Input: part model. Units: mm. Frame: model coordinates. Give positions to 0.01 mm unless a question says otherwise; leave off trailing zeros. Loops run counter-clockwise (first coordinate to the right, second up) from the corner with the lowest first, then second, coordinate; pieces in that order, holes last. Notation, with made-up numbers: (67.25, 79) - (79.25, 79) arc R14 cw to (79.25, 100) - close; hole circle Ø3 at (51, -23.5). An arc over 180 degrees is marked (long way). One line per question, with ' | ' between items. Start each with the question number.
from build123d import *

# Parameters (mm, degrees)
SKETCH_1_R                   = 31
EXTRUDE_1_DEPTH              = 6
SKETCH_3_R                   = 25
CUT_EXTRUDE_1_DEPTH          = 7
SKETCH_5_R                   = 31
SKETCH_5_R_2                 = 24
EXTRUDE_2_DEPTH              = 1
HOLE_WIZARD_M3_1_D           = 3.6
HOLE_WIZARD_M3_1_CSINK_D     = 6.3
HOLE_WIZARD_M3_1_CSINK_ANGLE = 90
PATTERN_CIRCULAR_1_COUNT     = 8
HOLE_WIZARD_M3_1_2_D         = 3.4
PATTERN_CIRCULAR_2_COUNT     = 8


with BuildPart() as part:
    # ｽｹｯﾁ1 → ﾎﾞｽ - 押し出し1 (new body)
    with BuildSketch(Plane.XY):
        Circle(SKETCH_1_R)
    extrude(amount=EXTRUDE_1_DEPTH)

    # ｽｹｯﾁ3 → ｶｯﾄ - 押し出し1 (cut, through all)
    with BuildSketch(Plane(origin=(0, 0, 0), x_dir=(-1, 0, 0), z_dir=(0, 0, -1))):
        Circle(SKETCH_3_R)
    extrude(amount=-CUT_EXTRUDE_1_DEPTH, mode=Mode.SUBTRACT)

    # ｽｹｯﾁ5 → ﾎﾞｽ - 押し出し2 (add)
    with BuildSketch(Plane(origin=(0, 0, 0), x_dir=(-1, 0, 0), z_dir=(0, 0, -1))):
        Circle(SKETCH_5_R)
        Circle(SKETCH_5_R_2, mode=Mode.SUBTRACT)
    extrude(amount=EXTRUDE_2_DEPTH)

    # Hole Wizard M3 _1 (through all)
    with Locations(Plane(origin=(0, 0, -1), x_dir=(-1, 0, 0), z_dir=(0, 0, -1))):
        with Locations((0, 27.5)):
            hole_wizard_m3_1 = CounterSinkHole(HOLE_WIZARD_M3_1_D / 2, HOLE_WIZARD_M3_1_CSINK_D / 2, counter_sink_angle=HOLE_WIZARD_M3_1_CSINK_ANGLE)

    # 円形ﾊﾟﾀｰﾝ1: Hole Wizard M3 _1 ×8 about axis
    pattern_circular_1_axis = Axis((0, 0, 0), (0, 0, 1))
    for i in range(1, PATTERN_CIRCULAR_1_COUNT):
        add(hole_wizard_m3_1.rotate(pattern_circular_1_axis, i * 360 / PATTERN_CIRCULAR_1_COUNT), mode=Mode.SUBTRACT)

    # Hole Wizard M3 _1 2 (through all)
    with Locations(Plane(origin=(0, 0, -1), x_dir=(-1, 0, 0), z_dir=(0, 0, -1))):
        with Locations((-10.52379439, 25.406687144)):
            hole_wizard_m3_1_2 = Hole(HOLE_WIZARD_M3_1_2_D / 2)

    # 円形ﾊﾟﾀｰﾝ2: Hole Wizard M3 _1 2 ×8 about axis
    pattern_circular_2_axis = Axis((0, 0, 0), (0, 0, 1))
    for i in range(1, PATTERN_CIRCULAR_2_COUNT):
        add(hole_wizard_m3_1_2.rotate(pattern_circular_2_axis, i * 360 / PATTERN_CIRCULAR_2_COUNT), mode=Mode.SUBTRACT)


solid = part.part
Q1. Section D-D, the plane y = 15. Output: boundary loops of the cut face in (x, z) (3 decimals).
Q2. First-contact query: pin 1 (6 mm diameter, centred on x = 0, y = 27.5, fed in from -Z); pin 2 (2 mm diameter, centred on y = -22, z = 1, fed in from +X); pin 3 (4 mm diameter, centred on x = -23, z = 3.5, fed in from +Y). Flat tips, straight axial feed; report the tip coordinate or a pass-through.
Q3. Section C-C, the plane z = 3.5. Count the separate pieces of the cut face and the enclosed holes in it, plus the area to 3 significant figures.
Q4. Draft query along Y for faces 1 (the face through (-0.234, 29.285, 3.215)), 2 (the face through (16.2, -18.2, -1)). Return one class per face: +Y half, -Y half, draft (parallel to the pull), parting line (faces both ways), or undercut.
Q5. Section A-A, the plane y = 0. Output: boundary loops of the cut face in (x, z).
Q6. Line query: L1, parallel to Y at x = 20, z = 4; L2, parallel to Y at x = 10, z = 1.5; L3, parallel to Y at x = -22.5, z = 1.25. Output: solid intervals per line, ascending. Write a range as from..to.
Solved:
1) outline: (-27.129, -1) - (-18.735, -1) - (-18.735, 0) - (-20, 0) - (-20, 6) - (-27.129, 6) - close; (18.735, -1) - (27.129, -1) - (27.129, 6) - (20, 6) - (20, 0) - (18.735, 0) - close
2) pin 1: stops at z = -0.85 | pin 2: stops at x = 22.8 | pin 3: stops at y = 22.8
3) separate pieces: 1 | enclosed holes: 17 | area: 902 mm²
4) face 1: undercut | face 2: draft
5) outline: (-31, -1) - (-30.65, -1) - (-29.3, 0.35) - (-29.3, 6) - (-31, 6) - close; (-25.7, 0.35) - (-24.35, -1) - (-24, -1) - (-24, 0) - (-25, 0) - (-25, 6) - (-25.7, 6) - close; (24, -1) - (24.35, -1) - (25.7, 0.35) - (25.7, 6) - (25, 6) - (25, 0) - (24, 0) - close; (29.3, 0.35) - (30.65, -1) - (31, -1) - (31, 6) - (29.3, 6) - close
6) L1: y = -23.69..-21.16, -17.73..-15, 15..17.73, 21.16..23.69 | L2: y = -29.34..-27.02, -23.79..-22.91, 22.91..23.79, 27.02..29.34 | L3: y = -21.32..-10.9, 10.9..21.32
